Can you work these out from the model? Positions are in its coordinate system, mm. A direction names the side the tool comes from. Coordinates: 2 decimals unless noted, no trailing zeros. Loops run counter-clockwise (first coordinate to the right, second up) from the corner with the lowest first, then second, coordinate; pieces in that order, holes last.
```python
from build123d import *

# Parameters (mm, degrees)
F0_W      = 96
F0_H      = 90
F1_DEPTH  = 18
F2_W      = 72
F2_H      = 38
F4_DEPTH  = 67
F6_DEPTH  = 38
F7_W      = 8
F7_H      = 12
F8_DEPTH  = 51.001
F10_DEPTH = 72.001
F11_W     = 20
F11_H     = 5
F12_DEPTH = 96
F13_W     = 46
F13_H     = 26
F14_DEPTH = 5
F16_DEPTH = 3
F17_W     = 3
F17_H     = 14
F18_DEPTH = 72
F19_R     = 2.99999


# Not quite as in the source:
# - a fillet or chamfer is up to 0.001 mm smaller than in the source, because OpenCascade refuses the exact size


with BuildPart() as f1:
    # F0 (on Top) → F1 (new body)
    with BuildSketch(Plane.XY):
        with Locations((48, 45)):
            Rectangle(F0_W, F0_H)
    extrude(amount=F1_DEPTH)

    # F2 (on face) → F4 (join, through all)
    with BuildSketch(Plane.XY.offset(18)):
        with Locations((48, 71)):
            Rectangle(F2_W, F2_H)
    extrude(amount=F4_DEPTH)

    # F5 (on face) → F6 (cut)
    with BuildSketch(Plane.XZ.offset(-52)):
        Polygon((84, 52), (84, 85), (51, 85), align=None)
    extrude(amount=-F6_DEPTH, mode=Mode.SUBTRACT)

    # F7 (on face) → F8 (cut, through all)
    with BuildSketch(Plane(origin=(12, 0, 0), x_dir=(0, -1, 0), z_dir=(-1, 0, 0))):
        with Locations((-64, 79)):
            Rectangle(F7_W, F7_H)
    extrude(amount=-F8_DEPTH, mode=Mode.SUBTRACT)

    # F9 (on face) → F10 (cut, through all)
    with BuildSketch(Plane(origin=(12, 0, 0), x_dir=(0, -1, 0), z_dir=(-1, 0, 0))):
        Polygon((-76, 85), (-90, 85), (-90, 40), align=None)
    extrude(amount=-F10_DEPTH, mode=Mode.SUBTRACT)

    # F11 (on face) → F12 (cut, through all)
    with BuildSketch(Plane.YZ.offset(96)):
        with Locations((32, 2.5)):
            Rectangle(F11_W, F11_H)
    extrude(amount=-F12_DEPTH, mode=Mode.SUBTRACT)

    # F13 (on face) → F14 (join)
    with BuildSketch(Plane.XY.offset(18)):
        with Locations((48, 32)):
            Rectangle(F13_W, F13_H)
        with BuildLine():
            Line((25, 19), (25, 45))
            ThreePointArc((25, 45), (12, 32), (25, 19))
        make_face()
        with BuildLine():
            ThreePointArc((71, 19), (84, 32), (71, 45))
            Line((71, 45), (71, 19))
        make_face()
    extrude(amount=F14_DEPTH)

    # F15 (on face) → F16 (cut)
    with BuildSketch(Plane.XY.offset(23)):
        with BuildLine():
            ThreePointArc((25, 38), (19, 32), (25, 26))
            Line((25, 26), (71, 26))
            ThreePointArc((71, 26), (77, 32), (71, 38))
            Line((71, 38), (25, 38))
        make_face()
    extrude(amount=-F16_DEPTH, mode=Mode.SUBTRACT)

    # F17 (on face) → F18 (cut, through all)
    with BuildSketch(Plane.YZ.offset(84)):
        with Locations((53.5, 25)):
            Rectangle(F17_W, F17_H)
    extrude(amount=-F18_DEPTH, mode=Mode.SUBTRACT)

    # F19 (radius 3 in the source; OpenCascade refuses exactly that, so slightly less here)
    f19_edges = [f1.edges().sort_by_distance(p)[0] for p in [
        (48, 19, 18),
        (48, 55, 18),
        (48, 55, 32),
        (90, 90, 18),
        (96, 0, 9),
        (96, 90, 9),
        (0, 90, 9),
        (0, 0, 9),
        (0, 45, 18),
        (96, 45, 18),
        (84, 72.5, 18),
        (48, 45, 18),
        (84, 32, 18),
        (12, 32, 18),
        (84, 90, 29),
    ]]
    fillet(f19_edges, radius=F19_R)


solid = f1.part
```
Item 1: We'd pull the mould along X, two halves only. Please class faces 5 (the face through (48, 32, 20)), 6 (the face through (49, 32, 5)), 7 (the face through (71, 65, 65)): +X half, -X half, draft (parallel to the pull), parting line (faces both ways), or undercut.
Results are:
face 5: undercut
face 6: draft
face 7: +X half
Item 2: Suppose I cut it at C-C, the plane z = 68. Please give me the cut outline in (x, y).
Results are:
outline: (12, 52) - (68, 52) - (68, 81.29) - (12, 81.29) - close
Item 3: I'm going to push flat-ended pins straight in: P1, Ø6, axis at y = 72.5, z = 26, coming from the -X side; P2, Ø9.5, axis at x = 25.5, z = 78, coming from the +Y side; P3, Ø8, axis at y = 45.5, z = 27.5, coming from the +X side; P4, Ø3, axis at x = 82.5, z = 20, coming from the -Y side. Where does each tip first touch, or does it pass through?
Results are:
P1: stops at x = 12
P2: stops at y = 79.66
P3: passes through
P4: stops at y = 22.91
Item 4: On a 3-axis mill with a long thin cutter (end or side, diameter ignored), from which of +Z, -Z, +X, -X, +Y, -Y can I reach the whole of each face in a straight line? I mean faces 1 (the face through (83.1, 89.14, 32.34)), 2 (the face through (48.97, 54.1, 18.86)), 3 (the face through (49, 22, 2)), 4 (the face through (37, 64, 73)). Say none if no direction works.
Results are:
face 1: +Z, +X, +Y
face 2: +X, -X
face 3: -Z, +X, -X
face 4: +Z, +X, -X
Item 5: I need wall thicknesses on line 1 along X through (y, z) = (57, 41); line 2 along Z through (x, y) = (59, 69.5); line 3 along Z through (x, y) = (15.5, 30.5). Which ranges of each line are inside material? Lowest first, please.
Results are:
line 1: x = 12 to 84
line 2: z = 0 to 77
line 3: z = 5 to 23
Item 6: Suppose I cut it at A-A, the plane y = 32. Please give me the cut outline in (x, z), plus the area to 3 significant figures.
Results are:
outline: (0, 5) - (96, 5) - (96, 15) arc R3 ccw to (93, 18) - (87, 18) arc R3 cw to (84, 21) - (84, 23) - (77, 23) - (77, 20) - (19, 20) - (19, 23) - (12, 23) - (12, 21) arc R3 cw to (9, 18) - (3, 18) arc R3 ccw to (0, 15) - close
area: 1,430 mm2
Item 7: Suppose I cut it at D-D, the plane y = 13. Please give me the cut outline in (x, z).
Results are:
outline: (0, 0) - (96, 0) - (96, 15) arc R3 ccw to (93, 18) - (3, 18) arc R3 ccw to (0, 15) - close
